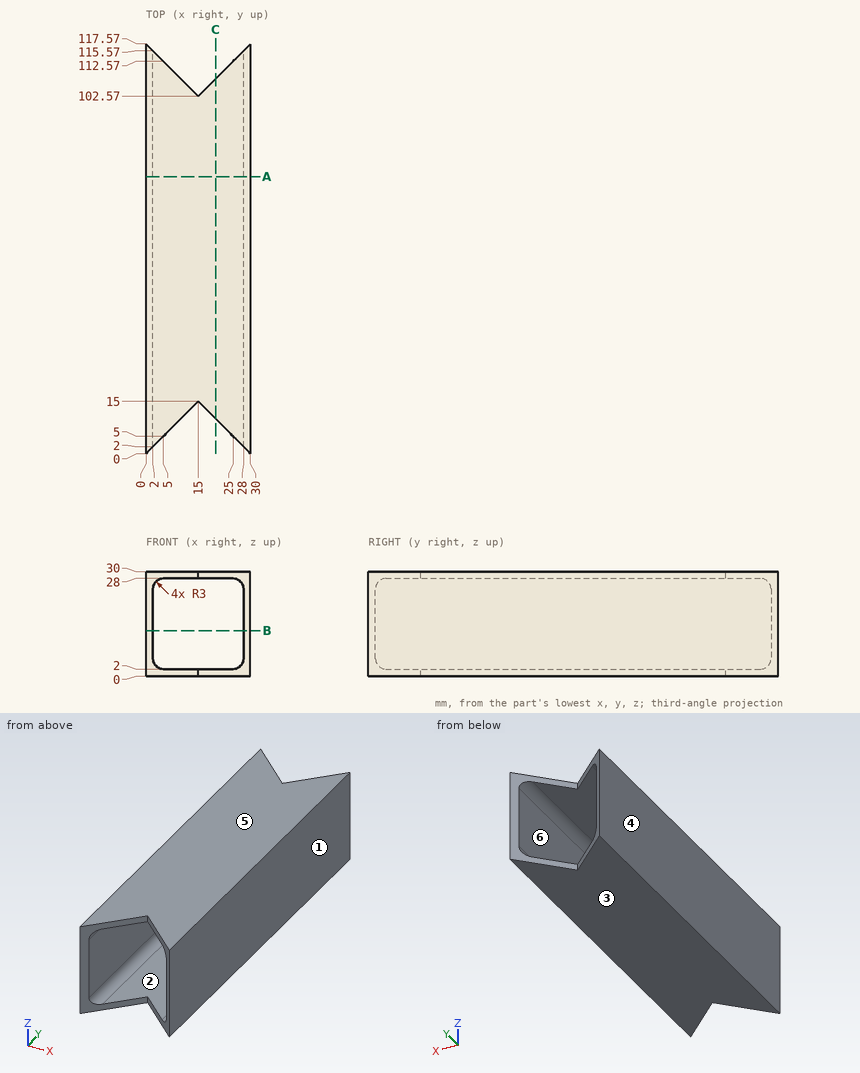
Design review of the part shown in the three views and the two pictorial views. Dimensions are in mm from the part's minimum x, y and z. A direction names the side the tool comes from. Round coordinates to 2 decimals unless told otherwise and drop trailing zeros. Loops run counter-clockwise (first coordinate to the right, second up) from the corner with the lowest first, then second, coordinate; pieces in that order, holes last. Notation, with made-up numbers: (-22.5, 26) - (20.5, 26) arc R7 cw to (20.5, 33) - close; hole circle Ø9 at (-9, 28.5). An arc over 180 degrees is marked (long way). Use one line per item in the form item = value.
1) Mouldability with a two-part tool opening along X and no side actions: class the marked faces 1, 2, 3 and 4 as pulls with the +X half, pulls with the -X half, needs draft (parallel to the pull), parting line crosses it, or undercut.
Solutions:
face_1 = pulls with the +X half
face_2 = undercut
face_3 = needs draft
face_4 = pulls with the -X half
2) We need section A-A on y = 79.5. Write out the cut boundary in (x, z), then the cut area to 3 significant figures.
Solutions:
outline = (0, 0) - (30, 0) - (30, 30) - (0, 30) - close; hole (2, 5) arc R3 ccw to (5, 2) - (25, 2) arc R3 ccw to (28, 5) - (28, 25) arc R3 ccw to (25, 28) - (5, 28) arc R3 ccw to (2, 25) - close
area = 232 mm2
3) Clearance check with a flat-ended pin moving along its axis: P1, Ø10, axis at x = 11, y = 35, coming from the -Z side. State where the tip first meets the part, or that it passes through.
Solutions:
P1 = 0
4) Tool access review of the marked faces 5 and 6: name each direction out of +Z, -Z, +X, -X, +Y, -Y from which nothing blocks a thin tool from reaching the whole face with its end or side.
Solutions:
face_5 = +Z, +X, -X, +Y, -Y
face_6 = +Y, -Y
5) We need section C-C on x = 20. Write out the cut boundary in (y, z).
Solutions:
outline = (10, 0) - (107.57, 0) - (107.57, 2) - (10, 2) - close; (10, 28) - (107.57, 28) - (107.57, 30) - (10, 30) - close
6) Wall thickness on probe 1 along X at (y, z) = (19, 11.75); probe 2 along X at (y, z) = (58, 27.5) (1 decimal): over which ranges is each line inside the solid? List them lowest first.
Solutions:
probe_1 = 0 to 2, 28 to 30
probe_2 = 0 to 3.3, 26.7 to 30
7) We need section B-B on z = 13. Write out the cut boundary in (x, y).
Solutions:
outline = (0, 0) - (2, 2) - (2, 115.57) - (0, 117.57) - close; (28, 2) - (30, 0) - (30, 117.57) - (28, 115.57) - close
